Verification items for the finished model (mm, model axes). Face numbers are marked on the shaded views. A direction names the side the tool comes from. Give positions to 0.01 mm unless a question says otherwise; leave off trailing zeros. Write each loop counter-clockwise with the first axis right and the second up, starting at its lowest first coordinate (ties: lowest second). Pieces come first, ordered by that corner, then holes. Notation, with made-up numbers: (80.25, 57) - (122.25, 57) arc R25 ccw to (122.25, 90) - close; hole circle Ø4 at (5.5, -20.5). An arc over 180 degrees is marked (long way). Put each result on its own line as item: value.
from build123d import *

# Parameters (mm, degrees)
SKETCH012_R     = 2.75
PAD007_DEPTH    = 3
SKETCH013_R     = 1.5
PAD008_DEPTH    = 10
POCKET004_DEPTH = 4


with BuildPart() as part:
    # Sketch012 → Pad007 (new body)
    with BuildSketch(Plane.XY):
        Circle(SKETCH012_R)
    extrude(amount=PAD007_DEPTH)

    # Sketch013 (on Face2 of Pad007) → Pad008 (join)
    with BuildSketch(Plane(origin=(0, 0, 0), x_dir=(1, 0, 0), z_dir=(0, 0, -1))):
        Circle(SKETCH013_R)
    extrude(amount=PAD008_DEPTH)

    # Sketch014 (on DatumPlane) → Pocket004 (cut)
    with BuildSketch(Plane.XY.offset(3)):
        Polygon((0.721688, -1.25), (1.443376, 0), (0.721688, 1.25), (-0.721688, 1.25), (-1.443376, 0), (-0.721688, -1.25), align=None)
    extrude(amount=-POCKET004_DEPTH, mode=Mode.SUBTRACT)


solid = part.part
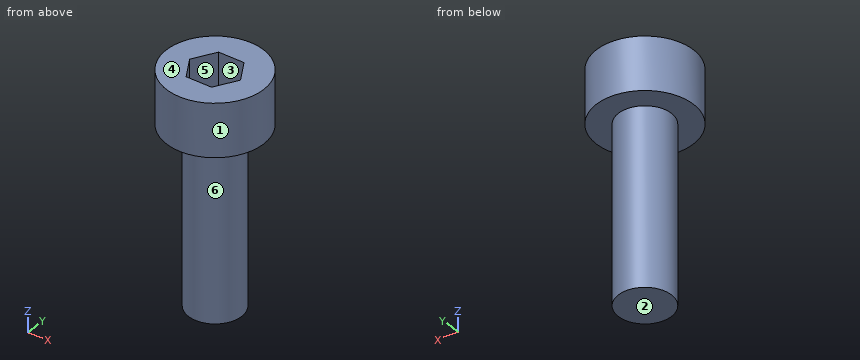
Q1. Go/stop test with flat-tipped pins: pin 1 Ø2 at (y, z) = (2, -7) entering from +X; pin 2 Ø2 at (x, y) = (-0.5, -0.5) entering from +Z; pin 3 Ø1 at (x, y) = (2, 0.5) entering from -Z; pin 4 Ø1 at (y, z) = (0.5, -2) entering from +X. Record where each tip stops, or that it passes through.
Answers follow:
pin 1: stops at x = 1.12
pin 2: stops at z = 3
pin 3: stops at z = 0
pin 4: stops at x = 1.5
Q2. Section check A-A, the plane z = -0.25. Record the cut outline in (x, y).
Answers follow:
outline: circle Ø3 at (0, 0); hole (-1.44, 0) - (-0.72, -1.25) - (0.72, -1.25) - (1.44, 0) - (0.72, 1.25) - (-0.72, 1.25) - close
Q3. Release check for a two-part mould opening along X. For the marked faces 1, 2 and 3 record: released by +X, released by -X, zero draft, split by the parting line, or undercut.
Answers follow:
face 1: split by the parting line
face 2: zero draft
face 3: undercut
Q4. Scan lines: line 1 along Z through (x, y) = (-0.1, 2.5); line 2 along X through (y, z) = (0.1, -2.5); line 3 along Z through (x, y) = (-0.2, -0.85). Record each from-to range of solid material in increasing order.
Answers follow:
line 1: z = 0 to 3
line 2: x = -1.5 to 1.5
line 3: z = -10 to -1
Q5. Section check C-C, the plane y = -0.65. Record the cut outline in (x, z).
Answers follow:
outline: (-2.67, 0) - (-1.35, 0) - (-1.35, -10) - (1.35, -10) - (1.35, 0) - (2.67, 0) - (2.67, 3) - (1.07, 3) - (1.07, -1) - (-1.07, -1) - (-1.07, 3) - (-2.67, 3) - close
Q6. Section check B-B, the plane x = 0. Record the cut outline in (y, z), plus the area to 3 significant figures.
Answers follow:
outline: (-2.75, 0) - (-1.5, 0) - (-1.5, -10) - (1.5, -10) - (1.5, 0) - (2.75, 0) - (2.75, 3) - (1.25, 3) - (1.25, -1) - (-1.25, -1) - (-1.25, 3) - (-2.75, 3) - close
area: 36.5 mm2
Q7. Set-up check for the marked faces 4, 5 and 6: record each of +Z, -Z, +X, -X, +Y, -Y from which the full face is reachable in a straight line by a thin tool's end or side.
Answers follow:
face 4: +Z, +X, -X, +Y, -Y
face 5: +Z
face 6: -Z
Q8. Section check D-D, the plane z = -2.5. Record the cut outline in (x, y), plus the area to 3 significant figures.
Answers follow:
outline: circle Ø3 at (0, 0)
area: 7.07 mm2
